Autodesk Inventor part; units mm, degrees
ref_plane "YZ Plane" through (0, 0, 0) normal (1, 0, 0) x (0, 1, 0)
ref_plane "XZ Plane" through (0, 0, 0) normal (0, 1, 0) x (-1, 0, 0)
ref_plane "XY Plane" through (0, 0, 0) normal (0, 0, 1) x (1, 0, 0)
sketch "Sketch3" plane through (0, 0, 0) normal (0, 1, 0) x (-1, 0, 0)
  line L0 (3.5626, 7.7011) -> (-78.4374, 7.7011)
  line L1 (-78.4374, -212.2989) -> (3.5626, -212.2989)
  line L2 (-84.4374, 13.7011) -> (9.5626, 13.7011)
  line L3 (9.5626, -212.2989) -> (3.5626, -212.2989)
  line L4 (-84.4374, -212.2989) -> (-78.4374, -212.2989)
  line L5 (-61.601, -206.2989) -> (-78.4374, -206.2989)
  line L6 (3.5626, -206.2989) -> (-61.601, -206.2989)
  line L7 (-84.4374, 13.7011) -> (-84.4374, -212.2989)
  line L8 (9.5626, 13.7011) -> (9.5626, -212.2989)
  line L9 (3.5626, -206.2989) -> (3.5626, 7.7011)
  line L10 (-78.4374, 7.7011) -> (-78.4374, -206.2989)
  point P0 (0, 0)
  dimension "d0" = 82
  dimension "d1" = 220
extrude "Extrusion1" add sketch "Sketch3" along normal blind 6 contours L9 L6 L5 L10 L0 | L4 L7 L2 L8 L3 L1
sketch "Sketch4" plane through (0, 6, 0) normal (0, 1, 0) x (1, 0, 0)
  line L0 (-9.5626, 212.2989) -> (-9.5626, -13.7011)
  line L1 (-9.5626, -13.7011) -> (-3.5626, -13.7011)
  line L2 (-9.5626, -13.7011) -> (84.4374, -13.7011)
  line L3 (-3.5626, -13.7011) -> (-3.5626, -7.6991)
  line L4 (-3.5626, -7.6991) -> (78.4374, -7.6991)
  line L5 (78.4374, -7.6991) -> (78.4374, 206.3009)
  line L6 (78.4374, 206.3009) -> (-3.5626, 206.3009)
  line L7 (-3.5626, 206.3009) -> (-3.5626, -7.6991)
  line L8 (84.4374, 212.2989) -> (-9.5626, 212.2989)
  line L9 (-9.5626, -13.7011) -> (84.4374, -13.7011)
  line L10 (84.4374, -13.7011) -> (84.4374, 212.2989)
  line L11 (84.4374, 212.2989) -> (-9.5626, 212.2989)
  line L12 (-9.5626, 212.2989) -> (-9.5626, -13.7011)
  point P0 (0, 0)
  dimension "d9" = 6
  dimension "d10" = 82
  dimension "d11" = 214
extrude "Extrusion2" add sketch "Sketch4" along normal blind 67
fillet "Fillet1" radius 3 8 edges at (84.4374, 36.5, -212.2989) (-9.5626, 36.5, -212.2989) (-9.5626, 36.5, 13.7011) (84.4374, 36.5, 13.7011) (37.4374, 0, 13.7011) (84.4374, 0, -99.2989) (-9.5626, 0, -99.2989) (37.4374, 0, -212.2989)
properties part number "Battery Box Bottom_3DPrint"
CAD build for the part. Positions are in the model's coordinates, mm. A direction names the side the tool comes from. Coordinates: 2 decimals unless noted, no trailing zeros. Loops run counter-clockwise (first coordinate to the right, second up) from the corner with the lowest first, then second, coordinate; pieces in that order, holes last. Notation, with made-up numbers: (54.25, -39.75) - (78.25, -39.75) arc R33 cw to (78.25, -0.75) - close; hole circle Ø8 at (82.5, 0.5). An arc over 180 degrees is marked (long way). Return JSON: item names as keys, results as strings.
1. Drop flat-ended pins along their axis: pin 1 (8 mm diameter, centred on x = 60.5, z = -19.5, fed in from -Y); pin 2 (24.5 mm diameter, centred on x = 36, z = -75, fed in from +Y). Give the stop position or say it passes through.
Result:
{"pin 1": "stops at y = 0", "pin 2": "stops at y = 6"}
2. 3-axis set-ups, long thin cutter, end or side, ignore diameter. For faces 1 (the flat face through (38, 39, -206.301)), 2 (the flat face through (37, 38, 13.701)): which of +Z, -Z, +X, -X, +Y, -Y reach the whole face in a straight line?
Result:
{"face 1": "+Y", "face 2": "+Z, +X, -X, +Y, -Y"}
3. Probe L1, parallel to Z at x = -1, y = 20; L2, parallel to X at y = 69, z = -170.5; L3, parallel to Y at x = 33.5, z = -13. List the from-to ranges inside material, lowest first. Write a range as from..to.
Result:
{"L1": "z = -212.3..-206.3, 7.7..13.7", "L2": "x = -9.56..-3.56, 78.44..84.44", "L3": "y = 0..6"}
4. Band-saw the part on C-C (x = 50.5). Give the cut face in (y, z), and give its area (3 significant figures).
Result:
{"outline": "(0, -209.3) arc R3 ccw to (3, -212.3) - (73, -212.3) - (73, -206.3) - (6, -206.3) - (6, 7.7) - (73, 7.7) - (73, 13.7) - (3, 13.7) arc R3 ccw to (0, 10.7) - close", "area": "2,160 mm2"}
5. Band-saw the part on B-B (z = -108.5). Give the cut face in (x, y), and give its area (3 significant figures).
Result:
{"outline": "(-9.56, 3) arc R3 ccw to (-6.56, 0) - (81.44, 0) arc R3 ccw to (84.44, 3) - (84.44, 73) - (78.44, 73) - (78.44, 6) - (-3.56, 6) - (-3.56, 73) - (-9.56, 73) - close", "area": "1,360 mm2"}
6. Band-saw the part on A-A (y = 23). Give the cut face in (x, z), and give its area (3 significant figures).
Result:
{"outline": "(-9.56, -209.3) arc R3 ccw to (-6.56, -212.3) - (81.44, -212.3) arc R3 ccw to (84.44, -209.3) - (84.44, 10.7) arc R3 ccw to (81.44, 13.7) - (-6.56, 13.7) arc R3 ccw to (-9.56, 10.7) - close; hole (-3.56, -206.3) - (78.44, -206.3) - (78.44, 7.7) - (-3.56, 7.7) - close", "area": "3,690 mm2"}
